The figure shows three views and two pictorial views of one solid part (mm, origin at its lowest corner). Answer the questions. A direction names the side the tool comes from. Coordinates: 2 decimals unless noted, no trailing zeros. Write each loop counter-clockwise with the first axis right and the second up, starting at its lowest first coordinate (ties: lowest second). Pieces come first, ordered by that corner, then holes.
Item 1: A tool of negligible diameter and unlimited length cuts with its end or side. For the marked faces 1 and 2, from which of +Z, -Z, +X, -X, +Y, -Y can it reach the whole face along a straight path? Write none if from no direction.
Item 2: Straight lines are drawn through the part: probe 1 along Z at (x, y) = (68, 40.5) (3 decimals); probe 2 along Y at (x, z) = (50, 99.25). For each, find the intervals that lie inside material, in ascending order.
Item 3: Section B-B (z = 57) is taken. Give the vertices of the cut face in (x, y) (3 decimals).
Item 4: Section C-C (y = 50) is taken. Give the vertices of the cut face in (x, z) (3 decimals), then the cut area to 3 significant figures.
Item 5: This flat-tipped pin is pushed along its axis until it touches: P1, Ø10, axis at x = 51, z = 90, coming from the -Y side (3 decimals). Where does it stop, or does it pass through?
Item 6: Section A-A (x = 50) is taken. Give the vertices of the cut face in (y, z) (3 decimals).
Item 7: Section D-D (x = 28.5) is taken. Give the vertices of the cut face in (y, z) (3 decimals), then the cut area to 3 significant figures.
Item 8: Determine the mould class of the marked faces 3, 4, 5 and 6 for opening direction X: released by +X, released by -X, zero draft, split by the parting line, or undercut.
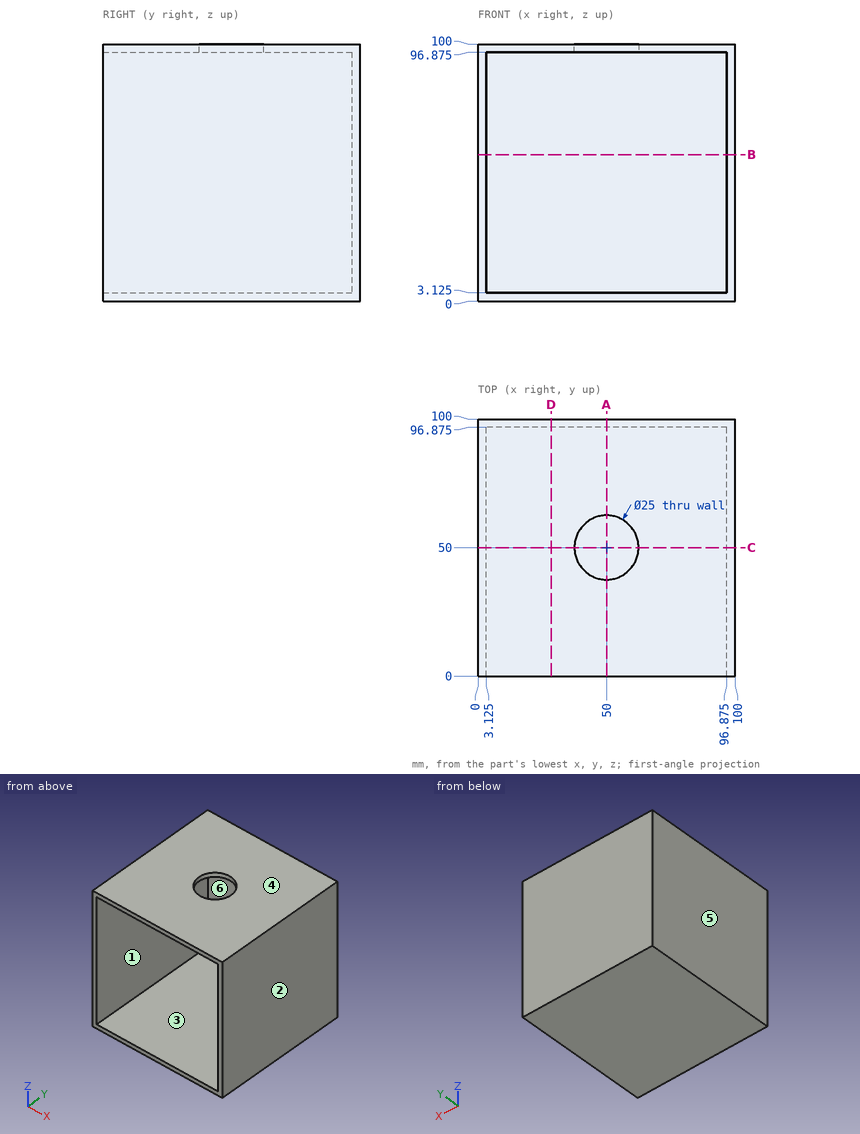
Established:
1. face 1: -Y
1. face 2: +Z, -Z, +X, +Y, -Y
2. probe 1: z = 0 to 3.125, 96.875 to 100
2. probe 2: y = 0 to 37.5, 62.5 to 100
3. outline: (0, 0) - (3.125, 0) - (3.125, 96.875) - (96.875, 96.875) - (96.875, 0) - (100, 0) - (100, 100) - (0, 100) - close
4. outline: (0, 0) - (100, 0) - (100, 100) - (62.5, 100) - (62.5, 96.875) - (96.875, 96.875) - (96.875, 3.125) - (3.125, 3.125) - (3.125, 96.875) - (37.5, 96.875) - (37.5, 100) - (0, 100) - close
4. area: 1,130 mm2
5. P1: stops at y = 96.875
6. outline: (0, 0) - (100, 0) - (100, 100) - (62.5, 100) - (62.5, 96.875) - (96.875, 96.875) - (96.875, 3.125) - (0, 3.125) - close; (0, 96.875) - (37.5, 96.875) - (37.5, 100) - (0, 100) - close
7. outline: (0, 0) - (100, 0) - (100, 100) - (0, 100) - (0, 96.875) - (96.875, 96.875) - (96.875, 3.125) - (0, 3.125) - close
7. area: 918 mm2
8. face 3: undercut
8. face 4: zero draft
8. face 5: released by -X
8. face 6: undercut
